from build123d import *

# Parameters (mm, degrees)
CHAMFER_1_SIZE = 1.6
CHAMFER_2_SIZE = 1


with BuildPart() as part:
    # Эскиз1 → Повернуть1 (revolve)
    with BuildSketch(Plane.XY, mode=Mode.PRIVATE) as revolve_1_sk:
        Polygon((3, -30.508474576), (12.5, -30.508474576), (12.5, -5.508474576), (7, -5.508474576), (7, 0), (8, 0), (8, 14.491525424), (3, 14.491525424), align=None)
    revolve(revolve_1_sk.sketch.rotate(Axis((0, 36.610169492, 0), (0, -1, 0)), 90), axis=Axis((0, 36.610169492, 0), (0, -1, 0)))

    # Фаска1
    chamfer_1_edges = [part.edges().sort_by_distance(p)[0] for p in [
        (0, -30.508474576, -12.5),
    ]]
    chamfer(chamfer_1_edges, length=CHAMFER_1_SIZE)

    # Фаска2
    chamfer_2_edges = [part.edges().sort_by_distance(p)[0] for p in [
        (0, 14.491525424, -8),
    ]]
    chamfer(chamfer_2_edges, length=CHAMFER_2_SIZE)


solid = part.part
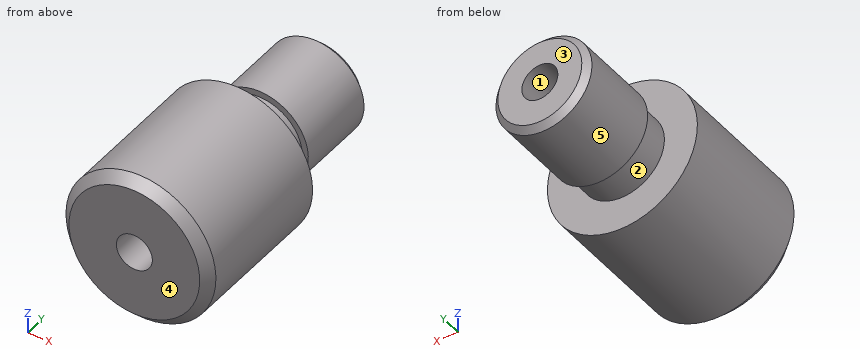
Source: CAD feature listing. Evaluate the final solid. Frame: model axes, mm. Face numbers are marked on the shaded views. A direction names the side the tool comes from. Round coordinates to 2 decimals unless told otherwise and drop trailing zeros. Loops run counter-clockwise (first coordinate to the right, second up) from the corner with the lowest first, then second, coordinate; pieces in that order, holes last. Notation, with made-up numbers: M 69.25,39.5 L 114.25,39.5 A12 ccw 114.25,58.5 Z; hole C 72,-2 d2. An arc over 180 degrees is marked long. Return JSON: item names as keys, results as strings. Group by question number.
1. Material intervals for line 1 along X through (y, z) = (-8, 0); line 2 along X through (y, z) = (-0.5, 0); line 3 along Z through (x, y) = (0.25, 1.5), sorted ascending. Write a range as from..to.
2. Section query B-B on z = 0. Output: boundary loops of the cut face in (x, y), and give its area (3 significant figures).
3. Section query D-D on y = 7. Output: boundary loops of the cut face in (x, z), and give its area (3 significant figures).
4. Reachability of the marked faces 4 and 5 from +Z, -Z, +X, -X, +Y, -Y: full face, straight path, thin tool, end or side. Return the list, or none.
5. Mould query, pull axis X, two halves, no side actions, for the marked faces 1, 2 and 3. Classes: released by +X, released by -X, zero draft, split by the parting line, or undercut.
6. Section query A-A on x = 0. Output: boundary loops of the cut face in (y, z).
7. Section query C-C on y = -8.5. Output: boundary loops of the cut face in (x, z), and give its area (3 significant figures).
8. Pin query (flat end, axial travel): pin 1 (2 mm diameter, centred on x = 2, y = 6, fed in from -Z); pin 2 (4 mm diameter, centred on y = 4.5, z = 4, fed in from -X); pin 3 (8 mm diameter, centred on y = -0.5, z = 1.5, fed in from -X). Return the tip coordinate at first contact, or that it passes through.
Checks:
{
 "1": {"line 1": "x = -12.5..-3, 3..12.5", "line 2": "x = -7..-3, 3..7", "line 3": "z = -8..-2.99, 2.99..8"},
 "2": {"outline": "M -12.5,-28.91 L -10.9,-30.51 L -3,-30.51 L -3,14.49 L -7,14.49 L -8,13.49 L -8,0 L -7,0 L -7,-5.51 L -12.5,-5.51 Z; M 3,-30.51 L 10.9,-30.51 L 12.5,-28.91 L 12.5,-5.51 L 7,-5.51 L 7,0 L 8,0 L 8,13.49 L 7,14.49 L 3,14.49 Z", "area": "660 mm²"},
 "3": {"outline": "C 0,0 d16; hole C 0,0 d6", "area": "173 mm²"},
 "4": {"face 4": "+Z, -Z, +X, -X, -Y", "face 5": "+Y"},
 "5": {"face 1": "undercut", "face 2": "split by the parting line", "face 3": "zero draft"},
 "6": {"outline": "M -30.51,-10.9 L -28.91,-12.5 L -5.51,-12.5 L -5.51,-7 L 0,-7 L 0,-8 L 13.49,-8 L 14.49,-7 L 14.49,-3 L -30.51,-3 Z; M -30.51,3 L 14.49,3 L 14.49,7 L 13.49,8 L 0,8 L 0,7 L -5.51,7 L -5.51,12.5 L -28.91,12.5 L -30.51,10.9 Z"},
 "7": {"outline": "C 0,0 d25; hole C 0,0 d6", "area": "463 mm²"},
 "8": {"pin 1": "stops at z = -7.94", "pin 2": "stops at x = -7.75", "pin 3": "stops at x = -8"}
}
